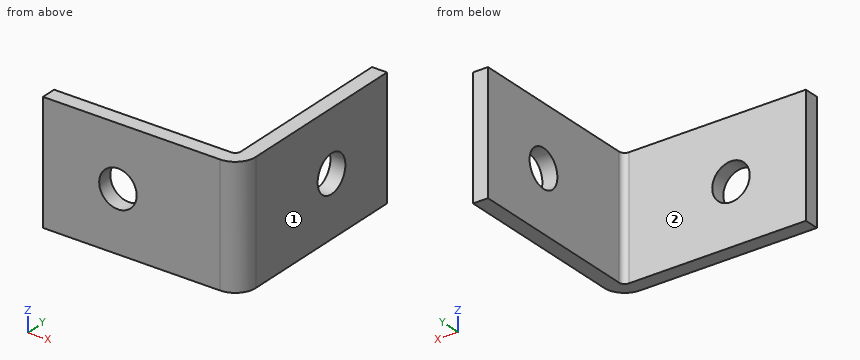
from build123d import *

# Parameters (mm, degrees)
CROQUIS2_W                      = 50
CROQUIS2_H                      = 16
CROQUIS2_R                      = 2.5
BRIDA_BASE1_DEPTH               = 2
PLIEGUE_START                   = -8
PLIEGUE_CROQUIZADO1_DEPTH       = 16
PLIEGUE_CROQUIZADO1_2_DEPTH     = 5.4999999
PLIEGUE_START_2                 = 2.5000001
PLIEGUE_CROQUIZADO1_3_DEPTH     = 5.4999999
PLIEGUE_START_3                 = -2.5000001
PLIEGUE_CROQUIZADO1_4_DEPTH     = 5.0000002
PLIEGUE_START_4                 = -0.627322451
PLIEGUE_CROQUIZADO1_5_OUTLINE_R = 2.5
PLIEGUE_CROQUIZADO1_5_DEPTH     = 2


with BuildPart() as part:
    # Brida base1: sheet metal written as solids
    # Croquis2 → Brida base1 (new body)
    with BuildSketch(Plane(origin=(0, 0, 0), x_dir=(1, 0, 0), z_dir=(0, 1, 0))):
        Rectangle(CROQUIS2_W, CROQUIS2_H)
        with Locations(Location((15, 0, 0), (0, 0, 270))):
            Circle(CROQUIS2_R, mode=Mode.SUBTRACT)
        with Locations(Location((-15, 0, 0), (0, 0, 270))):
            Circle(CROQUIS2_R, mode=Mode.SUBTRACT)
    extrude(amount=-BRIDA_BASE1_DEPTH)

    # Pliegue croquizado1: read off the stored shape, not the designer's step
    # Pliegue croquizado1 outline → Pliegue croquizado1 (cut)
    with BuildSketch(Plane.XY.offset(PLIEGUE_START)):
        with BuildLine():
            Line((25, 0), (1.271679947, 0))
            ThreePointArc((1.271679947, 0), (0.290344758, -1.443395312), (-1.363922451, -2))
            Line((-1.363922451, -2), (25, -2))
            Line((25, -2), (25, 0))
        make_face()
    extrude(amount=PLIEGUE_CROQUIZADO1_DEPTH, mode=Mode.SUBTRACT)

    # Pliegue croquizado1 2 outline → Pliegue croquizado1 2 (add)
    with BuildSketch(Plane.XY.offset(PLIEGUE_START)):
        with BuildLine():
            Line((-0.627322451, 24.372677549), (-0.627322451, 0.7366))
            ThreePointArc((-0.627322451, 0.7366), (-0.843067596, 0.215745145), (-1.363922451, 0))
            Line((-1.363922451, 0), (1.271679947, 0))
            ThreePointArc((1.271679947, 0), (1.347310579, 0.364854094), (1.372677549, 0.7366))
            Line((1.372677549, 0.7366), (1.372677549, 24.372677549))
            Line((1.372677549, 24.372677549), (-0.627322451, 24.372677549))
        make_face()
    extrude(amount=PLIEGUE_CROQUIZADO1_2_DEPTH)

    # Pliegue croquizado1 3 outline → Pliegue croquizado1 3 (add)
    with BuildSketch(Plane.XY.offset(PLIEGUE_START_2)):
        with BuildLine():
            Line((-0.627322451, 24.372677549), (-0.627322451, 0.7366))
            ThreePointArc((-0.627322451, 0.7366), (-0.843067596, 0.215745145), (-1.363922451, 0))
            Line((-1.363922451, 0), (1.271679947, 0))
            ThreePointArc((1.271679947, 0), (1.347310579, 0.364854094), (1.372677549, 0.7366))
            Line((1.372677549, 0.7366), (1.372677549, 24.372677549))
            Line((1.372677549, 24.372677549), (-0.627322451, 24.372677549))
        make_face()
    extrude(amount=PLIEGUE_CROQUIZADO1_3_DEPTH)

    # Pliegue croquizado1 4 outline → Pliegue croquizado1 4 (add)
    with BuildSketch(Plane.XY.offset(PLIEGUE_START_3)):
        with BuildLine():
            Line((-0.627322451, 24.372677549), (-0.627322451, 0.7366))
            ThreePointArc((-0.627322451, 0.7366), (-0.843067596, 0.215745145), (-1.363922451, 0))
            Line((-1.363922451, 0), (1.271679947, 0))
            ThreePointArc((1.271679947, 0), (1.347310579, 0.364854094), (1.372677549, 0.7366))
            Line((1.372677549, 0.7366), (1.372677549, 24.372677549))
            Line((1.372677549, 24.372677549), (-0.627322451, 24.372677549))
        make_face()
    extrude(amount=PLIEGUE_CROQUIZADO1_4_DEPTH)

    # Pliegue croquizado1 5 outline → Pliegue croquizado1 5 (cut)
    with BuildSketch(Plane.YZ.offset(PLIEGUE_START_4)):
        with Locations((14.372677549, 0)):
            Circle(PLIEGUE_CROQUIZADO1_5_OUTLINE_R)
    extrude(amount=PLIEGUE_CROQUIZADO1_5_DEPTH, mode=Mode.SUBTRACT)


solid = part.part
For this review, take the finished solid that the model builds, in its own axes (mm). Face numbers are marked on the shaded views. A direction names the side the tool comes from. Round coordinates to 2 decimals unless told otherwise and drop trailing zeros. Order: outer loops, then holes, each group sorted by start corner. A loop starts at its lowest first (then second) coordinate and runs counter-clockwise, first axis right, second up. Notation, with made-up numbers: (29.25, 73) -> (82.25, 73) arc R18 cw to (82.25, 100) -> close; hole circle Ø9 at (41, 62.5). An arc over 180 degrees is marked (long way). Write item = value, one per line. Start each with the question number.
1) To check wall thickness, follow line 1 (X direction, y = 22.25, z = -5); line 2 (X direction, y = -1.1, z = 0); line 3 (Y direction, x = -13.5, z = -5). State the ranges of each line that lie inside material, in increasing order. Write a range as from..to.
2) Tool access review of the marked faces 1 and 2: name each direction out of +Z, -Z, +X, -X, +Y, -Y from which nothing blocks a thin tool from reaching the whole face with its end or side.
3) Take a section at B-B on z = 0. State the section outline as (x, y) points, plus the area to 3 significant figures.
4) Take a section at D-D on y = 17.5. State the section outline as (x, z) points.
5) Take a section at C-C on z = -4.75. State the section outline as (x, y) points.
6) Take a section at A-A on x = -15. State the section outline as (y, z) points, plus the area to 3 significant figures.
7) Insertion check: pin 1 (1 mm diameter, centred on y = 11.5, z = 6, fed in from -X); pin 2 (4 mm diameter, centred on x = -9, z = -5, fed in from +Y). Each pin has a flat end and moves straight along its axis. Give the tip position at first contact, or say it passes through.
Verdict:
q1.line_1 = -0.63..1.37
q1.line_2 = -25..-17.5, -12.5..0.66
q1.line_3 = -2..0
q2.face_1 = +Z, -Z, +X, +Y, -Y
q2.face_2 = +Z, -Z, -X, +Y
q3.outline = (-25, -2) -> (-17.5, -2) -> (-17.5, 0) -> (-25, 0) -> close; (-12.5, -2) -> (-1.36, -2) arc R2.74 ccw to (1.37, 0.74) -> (1.37, 11.87) -> (-0.63, 11.87) -> (-0.63, 0.74) arc R0.74 cw to (-1.36, 0) -> (-12.5, 0) -> close; (-0.63, 16.87) -> (1.37, 16.87) -> (1.37, 24.37) -> (-0.63, 24.37) -> close
q3.area = 80.0 mm2
q4.outline = (-0.63, -8) -> (1.37, -8) -> (1.37, 8) -> (-0.63, 8) -> close
q5.outline = (-25, -2) -> (-1.36, -2) arc R2.74 ccw to (1.37, 0.74) -> (1.37, 24.37) -> (-0.63, 24.37) -> (-0.63, 0.74) arc R0.74 cw to (-1.36, 0) -> (-25, 0) -> close
q6.outline = (-2, -8) -> (0, -8) -> (0, -2.5) -> (-2, -2.5) -> close; (-2, 2.5) -> (0, 2.5) -> (0, 8) -> (-2, 8) -> close
q6.area = 22.0 mm2
q7.pin_1 = -0.63
q7.pin_2 = 0
